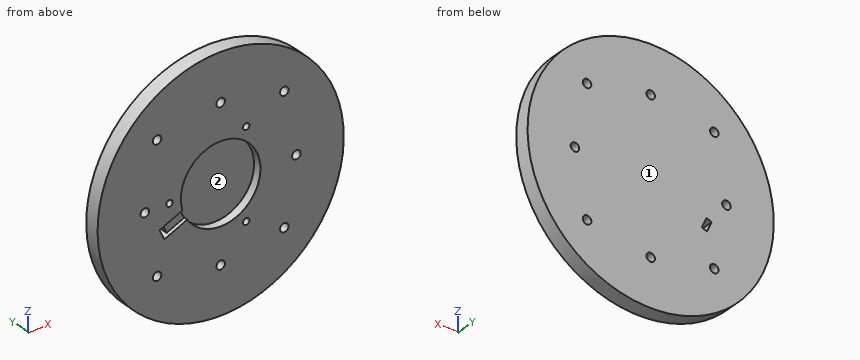
from build123d import *

# Parameters (mm, degrees)
SKETCH2_R           = 65
BOSS_EXTRUDE1_DEPTH = 8
SKETCH3_R           = 21
CUT_EXTRUDE1_DEPTH  = 4.5
SKETCH4_R           = 2.25
CUT_EXTRUDE2_DEPTH  = 93.271338995
SKETCH5_R           = 2.25
CUT_EXTRUDE3_DEPTH  = 93.271338995
PATH_TRENCH_DEPTH   = 2
CDG_R               = 1.7
CDG_CUT_DEPTH       = 6
CUT_EXTRUDE4_DEPTH  = 93.271338995


with BuildPart() as part:
    # Sketch2 → Boss-Extrude1 (new body)
    with BuildSketch(Plane(origin=(0, 0, 0), x_dir=(1, 0, 0), z_dir=(0, 1, 0))):
        with Locations(Location((0, 0, 0), (0, 0, 270))):
            Circle(SKETCH2_R)
    extrude(amount=BOSS_EXTRUDE1_DEPTH)

    # Sketch3 → Cut-Extrude1 (cut)
    with BuildSketch(Plane.XZ):
        with Locations(Location((0, 0, 0), (0, 0, 270))):
            Circle(SKETCH3_R)
    extrude(amount=-CUT_EXTRUDE1_DEPTH, mode=Mode.SUBTRACT)

    # Sketch4 → Cut-Extrude2 (cut, through all)
    with BuildSketch(Plane(origin=(0, 8, 0), x_dir=(1, 0, 0), z_dir=(0, 1, 0))):
        with Locations(Location((-40, 0, 0), (0, 0, 270))):
            Circle(SKETCH4_R)
        with Locations(Location((0, 40, 0), (0, 0, 270))):
            Circle(SKETCH4_R)
        with Locations(Location((40, 0, 0), (0, 0, 270))):
            Circle(SKETCH4_R)
        with Locations(Location((0, -40, 0), (0, 0, 270))):
            Circle(SKETCH4_R)
    extrude(amount=-CUT_EXTRUDE2_DEPTH, mode=Mode.SUBTRACT)

    # Sketch5 → Cut-Extrude3 (cut, through all)
    with BuildSketch(Plane(origin=(0, 8, 0), x_dir=(1, 0, 0), z_dir=(0, 1, 0))):
        with Locations(Location((-33.587572106, 33.587572106, 0), (0, 0, 270))):
            Circle(SKETCH5_R)
        with Locations(Location((33.587572106, 33.587572106, 0), (0, 0, 270))):
            Circle(SKETCH5_R)
        with Locations(Location((33.587572106, -33.587572106, 0), (0, 0, 270))):
            Circle(SKETCH5_R)
        with Locations(Location((-33.587572106, -33.587572106, 0), (0, 0, 270))):
            Circle(SKETCH5_R)
    extrude(amount=-CUT_EXTRUDE3_DEPTH, mode=Mode.SUBTRACT)

    # Sketch6 → path_trench (cut)
    with BuildSketch(Plane.XZ):
        Polygon((-29.480467623, -10.045000187), (-27.007252724, -15.511553769), (-16.07414556, -10.565123971), (-18.547360459, -5.098570389), align=None)
    extrude(amount=-PATH_TRENCH_DEPTH, mode=Mode.SUBTRACT)

    # CDG → CDG_CUT (cut)
    with BuildSketch(Plane.XZ):
        with Locations(Location((-27, 0, 0), (0, 0, 270))):
            Circle(CDG_R)
        with Locations(Location((13.5, 23.382685902, 0), (0, 0, 270))):
            Circle(CDG_R)
        with Locations(Location((13.5, -23.382685902, 0), (0, 0, 270))):
            Circle(CDG_R)
    extrude(amount=-CDG_CUT_DEPTH, mode=Mode.SUBTRACT)

    # Sketch7 → Cut-Extrude4 (cut, through all)
    with BuildSketch(Plane.XZ):
        Polygon((-29.480467623, -10.045000187), (-32.213744414, -11.281607636), (-29.740529515, -16.748161218), (-27.007252724, -15.511553769), align=None)
    extrude(amount=-CUT_EXTRUDE4_DEPTH, mode=Mode.SUBTRACT)


solid = part.part
Can you work these out from the model? Positions are in its coordinate system, mm. Face numbers are marked on the shaded views. Give positions to 0.01 mm unless a question says otherwise; leave off trailing zeros. Loops run counter-clockwise (first coordinate to the right, second up) from the corner with the lowest first, then second, coordinate; pieces in that order, holes last. Notation, with made-up numbers: (61, 42.5) -> (108, 42.5) arc R16 cw to (108, 46.5) -> close; hole circle Ø4 at (67.25, 54.25). An arc over 180 degrees is marked (long way). Return JSON: item names as keys, results as strings.
Q1. We'd pull the mould along Z, two halves only. Please class the marked faces 1 and 2: released by +Z, released by -Z, zero draft, split by the parting line, or undercut.
Checks:
{"face 1": "zero draft", "face 2": "undercut"}
Q2. I want a section at B-B, the plane z = -40. List the corners of the cut face in (x, y) for me.
Checks:
{"outline": "(-51.23, 0) -> (-2.25, 0) -> (-2.25, 8) -> (-51.23, 8) -> close; (2.25, 0) -> (51.23, 0) -> (51.23, 8) -> (2.25, 8) -> close"}
Q3. For pin 1 Ø4 at (x, y) = (-41.5, 2.5) entering from -Z; pin 2 Ø2.5 at (x, z) = (40, 0) entering from -Y; pin 3 Ø1 at (x, z) = (-27, 0) entering from -Y; pin 4 Ø10 at (x, z) = (2, 2.5) entering from -Y, each with a flat end and sliding along its axis, tell me the tip position at first contact or that it passes through.
Checks:
{"pin 1": "stops at z = -51.62", "pin 2": "passes through", "pin 3": "stops at y = 6", "pin 4": "stops at y = 4.5"}
Q4. I want a section at D-D, the plane z = 53. List the corners of the cut face in (x, y) for me.
Checks:
{"outline": "(-37.63, 0) -> (37.63, 0) -> (37.63, 8) -> (-37.63, 8) -> close"}
Q5. I need wall thicknesses on probe 1 along X at (y, z) = (2, 0); probe 2 along X at (y, z) = (4.5, -32); probe 3 along Z at (x, y) = (4, 2.5). Which ranges of each line are inside material? Lowest first, please.
Checks:
{"probe 1": "x = -65 to -42.25, -37.75 to -28.7, -25.3 to -21, 21 to 37.75, 42.25 to 65", "probe 2": "x = -56.58 to -35.18, -31.99 to 31.99, 35.18 to 56.58", "probe 3": "z = -64.88 to -20.62, 20.62 to 64.88"}
Q6. I want a section at A-A, the plane x = 0. List the corners of the cut face in (y, z) for me.
Checks:
{"outline": "(0, -65) -> (8, -65) -> (8, -42.25) -> (0, -42.25) -> close; (0, -37.75) -> (8, -37.75) -> (8, 37.75) -> (0, 37.75) -> (0, 21) -> (4.5, 21) -> (4.5, -21) -> (0, -21) -> close; (0, 42.25) -> (8, 42.25) -> (8, 65) -> (0, 65) -> close"}
Q7. I want a section at C-C, the plane x = 40. List the corners of the cut face in (y, z) for me, then the cut area to 3 significant figures.
Checks:
{"outline": "(0, -51.23) -> (8, -51.23) -> (8, -2.25) -> (0, -2.25) -> close; (0, 2.25) -> (8, 2.25) -> (8, 51.23) -> (0, 51.23) -> close", "area": "784 mm2"}
